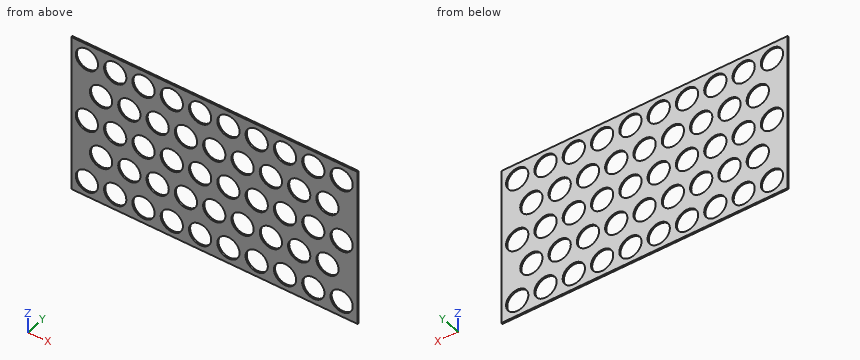
from build123d import *

# Parameters (mm, degrees)
SKETCH1_W               = 228.6
SKETCH1_H               = 127
BOSS_EXTRUDE1_DEPTH     = 1.27
CUT_EXTRUDE1_DEPTH      = 176.706526426
CUT_EXTRUDE1_DEPTH_BACK = 176.706526426
SKETCH2_R               = 8.89


with BuildPart() as part:
    # Sketch1 → Boss-Extrude1 (new body)
    with BuildSketch(Plane(origin=(0, 0, 0), x_dir=(1, 0, 0), z_dir=(0, 1, 0))):
        with Locations((26.414806677, -41.716508736)):
            Rectangle(SKETCH1_W, SKETCH1_H)
    extrude(amount=BOSS_EXTRUDE1_DEPTH)

    # Sketch2 → Cut-Extrude1 (cut, two sides: drawn at the far end of the back side and taken through both)
    with BuildSketch(Plane(origin=(0, 1.27, 0), x_dir=(1, 0, 0), z_dir=(0, 1, 0)).offset(-CUT_EXTRUDE1_DEPTH_BACK)):
        with Locations(Location((128.014806677, 9.083491264, 0), (0, 0, 270))):
            Circle(SKETCH2_R)
        with Locations(Location((105.408806677, 9.083491264, 0), (0, 0, 270))):
            Circle(SKETCH2_R)
        with Locations(Location((82.802806677, 9.083491264, 0), (0, 0, 270))):
            Circle(SKETCH2_R)
        with Locations(Location((60.196806677, 9.083491264, 0), (0, 0, 270))):
            Circle(SKETCH2_R)
        with Locations(Location((37.590806677, 9.083491264, 0), (0, 0, 270))):
            Circle(SKETCH2_R)
        with Locations(Location((14.984806677, 9.083491264, 0), (0, 0, 270))):
            Circle(SKETCH2_R)
        with Locations(Location((-7.621193323, 9.083491264, 0), (0, 0, 270))):
            Circle(SKETCH2_R)
        with Locations(Location((-30.227193323, 9.083491264, 0), (0, 0, 270))):
            Circle(SKETCH2_R)
        with Locations(Location((-52.833193323, 9.083491264, 0), (0, 0, 270))):
            Circle(SKETCH2_R)
        with Locations(Location((-75.439193323, 9.083491264, 0), (0, 0, 270))):
            Circle(SKETCH2_R)
        with Locations(Location((128.014806677, -41.716508736, 0), (0, 0, 270))):
            Circle(SKETCH2_R)
        with Locations(Location((128.014806677, -92.516508736, 0), (0, 0, 270))):
            Circle(SKETCH2_R)
        with Locations(Location((105.408806677, -41.716508736, 0), (0, 0, 270))):
            Circle(SKETCH2_R)
        with Locations(Location((105.408806677, -92.516508736, 0), (0, 0, 270))):
            Circle(SKETCH2_R)
        with Locations(Location((82.802806677, -41.716508736, 0), (0, 0, 270))):
            Circle(SKETCH2_R)
        with Locations(Location((82.802806677, -92.516508736, 0), (0, 0, 270))):
            Circle(SKETCH2_R)
        with Locations(Location((60.196806677, -41.716508736, 0), (0, 0, 270))):
            Circle(SKETCH2_R)
        with Locations(Location((60.196806677, -92.516508736, 0), (0, 0, 270))):
            Circle(SKETCH2_R)
        with Locations(Location((37.590806677, -41.716508736, 0), (0, 0, 270))):
            Circle(SKETCH2_R)
        with Locations(Location((37.590806677, -92.516508736, 0), (0, 0, 270))):
            Circle(SKETCH2_R)
        with Locations(Location((14.984806677, -41.716508736, 0), (0, 0, 270))):
            Circle(SKETCH2_R)
        with Locations(Location((14.984806677, -92.516508736, 0), (0, 0, 270))):
            Circle(SKETCH2_R)
        with Locations(Location((-7.621193323, -41.716508736, 0), (0, 0, 270))):
            Circle(SKETCH2_R)
        with Locations(Location((-7.621193323, -92.516508736, 0), (0, 0, 270))):
            Circle(SKETCH2_R)
        with Locations(Location((-30.227193323, -41.716508736, 0), (0, 0, 270))):
            Circle(SKETCH2_R)
        with Locations(Location((-30.227193323, -92.516508736, 0), (0, 0, 270))):
            Circle(SKETCH2_R)
        with Locations(Location((-52.833193323, -41.716508736, 0), (0, 0, 270))):
            Circle(SKETCH2_R)
        with Locations(Location((-52.833193323, -92.516508736, 0), (0, 0, 270))):
            Circle(SKETCH2_R)
        with Locations(Location((-75.439193323, -41.716508736, 0), (0, 0, 270))):
            Circle(SKETCH2_R)
        with Locations(Location((-75.439193323, -92.516508736, 0), (0, 0, 270))):
            Circle(SKETCH2_R)
        with Locations(Location((116.711806677, -16.316508736, 0), (0, 0, 270))):
            Circle(SKETCH2_R)
        with Locations(Location((116.711806677, -67.116508736, 0), (0, 0, 270))):
            Circle(SKETCH2_R)
        with Locations(Location((94.105806677, -16.316508736, 0), (0, 0, 270))):
            Circle(SKETCH2_R)
        with Locations(Location((94.105806677, -67.116508736, 0), (0, 0, 270))):
            Circle(SKETCH2_R)
        with Locations(Location((71.499806677, -16.316508736, 0), (0, 0, 270))):
            Circle(SKETCH2_R)
        with Locations(Location((71.499806677, -67.116508736, 0), (0, 0, 270))):
            Circle(SKETCH2_R)
        with Locations(Location((48.893806677, -16.316508736, 0), (0, 0, 270))):
            Circle(SKETCH2_R)
        with Locations(Location((48.893806677, -67.116508736, 0), (0, 0, 270))):
            Circle(SKETCH2_R)
        with Locations(Location((26.287806677, -16.316508736, 0), (0, 0, 270))):
            Circle(SKETCH2_R)
        with Locations(Location((26.287806677, -67.116508736, 0), (0, 0, 270))):
            Circle(SKETCH2_R)
        with Locations(Location((3.681806677, -16.316508736, 0), (0, 0, 270))):
            Circle(SKETCH2_R)
        with Locations(Location((3.681806677, -67.116508736, 0), (0, 0, 270))):
            Circle(SKETCH2_R)
        with Locations(Location((-18.924193323, -16.316508736, 0), (0, 0, 270))):
            Circle(SKETCH2_R)
        with Locations(Location((-18.924193323, -67.116508736, 0), (0, 0, 270))):
            Circle(SKETCH2_R)
        with Locations(Location((-41.530193323, -16.316508736, 0), (0, 0, 270))):
            Circle(SKETCH2_R)
        with Locations(Location((-41.530193323, -67.116508736, 0), (0, 0, 270))):
            Circle(SKETCH2_R)
        with Locations(Location((-64.136193323, -16.316508736, 0), (0, 0, 270))):
            Circle(SKETCH2_R)
        with Locations(Location((-64.136193323, -67.116508736, 0), (0, 0, 270))):
            Circle(SKETCH2_R)
    extrude(amount=CUT_EXTRUDE1_DEPTH + CUT_EXTRUDE1_DEPTH_BACK, mode=Mode.SUBTRACT)


solid = part.part
Build history of the part. All positions in model axes, mm. Round coordinates to 2 decimals unless told otherwise and drop trailing zeros. Loops run counter-clockwise (first coordinate to the right, second up) from the corner with the lowest first, then second, coordinate; pieces in that order, holes last. Notation, with made-up numbers: (-22.75, 30) -> (5.25, 30) arc R30 cw to (5.25, 59) -> close; hole circle Ø3 at (-9, -40). An arc over 180 degrees is marked (long way). Answer in a Markdown table with one row per item.
Item 1: Saw through at C-C (y = 0.45). State how many separate pieces and enclosed holes the cut face has, and give its area (3 significant figures).
Answers below:
| item | result |
|---|---|
| separate pieces | 1 |
| enclosed holes | 48 |
| area | 17,100 mm² |
Item 2: Drill centre lines: L1, parallel to Z at x = -7, y = 0.3; L2, parallel to Z at x = -52, y = 0.2; L3, parallel to Z at x = -24.5, y = 0.35. Where is each one in solid material? Low to high. Write a range as [from, to].
Answers below:
| item | result |
|---|---|
| L1 | z = [-21.78, -17.95], [-0.22, 32.85], [50.58, 83.65], [101.38, 105.22] |
| L2 | z = [-21.78, -17.93], [-0.23, 32.87], [50.57, 83.67], [101.37, 105.22] |
| L3 | z = [-21.78, -15.88], [-2.28, 9.39], [23.24, 34.92], [48.52, 60.19], [74.04, 85.72], [99.32, 105.22] |
Item 3: Saw through at A-A (x = 123.5). Write the cut outline in (y, z), and give its area (3 significant figures).
Answers below:
| item | result |
|---|---|
| outline | (0, -21.78) -> (1.27, -21.78) -> (1.27, -16.74) -> (0, -16.74) -> close; (0, -1.43) -> (1.27, -1.43) -> (1.27, 10.58) -> (0, 10.58) -> close; (0, 22.06) -> (1.27, 22.06) -> (1.27, 34.06) -> (0, 34.06) -> close; (0, 49.37) -> (1.27, 49.37) -> (1.27, 61.38) -> (0, 61.38) -> close; (0, 72.86) -> (1.27, 72.86) -> (1.27, 84.86) -> (0, 84.86) -> close; (0, 100.17) -> (1.27, 100.17) -> (1.27, 105.22) -> (0, 105.22) -> close |
| area | 73.8 mm² |
Item 4: Pin check, flat tip, straight feed: pin 1 (4 mm diameter, centred on x = 16.5, z = 64.5, fed in from -Y). Stop position of the tip, or through.
Answers below:
| item | result |
|---|---|
| pin 1 | stops at y = 0 |
Item 5: Saw through at B-B (x = 33). Write the cut outline in (y, z).
Answers below:
| item | result |
|---|---|
| outline | (0, -21.78) -> (1.27, -21.78) -> (1.27, -16.7) -> (0, -16.7) -> close; (0, -1.47) -> (1.27, -1.47) -> (1.27, 10.49) -> (0, 10.49) -> close; (0, 22.15) -> (1.27, 22.15) -> (1.27, 34.1) -> (0, 34.1) -> close; (0, 49.33) -> (1.27, 49.33) -> (1.27, 61.29) -> (0, 61.29) -> close; (0, 72.95) -> (1.27, 72.95) -> (1.27, 84.9) -> (0, 84.9) -> close; (0, 100.13) -> (1.27, 100.13) -> (1.27, 105.22) -> (0, 105.22) -> close |
